Build history of the part. All positions in model axes, mm. A direction names the side the tool comes from. Round coordinates to 2 decimals unless told otherwise and drop trailing zeros. Loops run counter-clockwise (first coordinate to the right, second up) from the corner with the lowest first, then second, coordinate; pieces in that order, holes last.
from build123d import *

# Parameters (mm, degrees)
F1_DEPTH = 64.77
F4_DEPTH = 2.54
F5_DEPTH = 2.54
F6_R     = 2.667
F6_R_2   = 19.05
F7_DEPTH = 70.613
F9_DEPTH = 70.613


with BuildPart() as f1:
    # F0 (on Right) → F1 (new body)
    with BuildSketch(Plane.YZ):
        with BuildLine():
            Line((-58.708991, 56.24623), (-61.375991, 56.24623))
            Line((-61.375991, 56.24623), (-61.375991, -11.69877))
            Line((-61.375991, -11.69877), (-129.320991, -11.69877))
            Line((-129.320991, -11.69877), (-129.320991, -14.36577))
            Line((-129.320991, -14.36577), (-61.248991, -14.36577))
            ThreePointArc((-61.248991, -14.36577), (-59.45294, -13.621821), (-58.708991, -11.82577))
            Line((-58.708991, -11.82577), (-58.708991, 56.24623))
        make_face()
    extrude(amount=F1_DEPTH)

    # F3 (on face) → F4 (join)
    with BuildSketch(Plane(origin=(0, 0, 0), x_dir=(0, -1, 0), z_dir=(-1, 0, 0))):
        with BuildLine():
            Line((77.885991, -11.69877), (61.375991, 14.97123))
            Line((61.375991, 14.97123), (61.375991, -7.88877))
            ThreePointArc((61.375991, -7.88877), (62.491914, -10.582847), (65.185991, -11.69877))
            Line((65.185991, -11.69877), (77.885991, -11.69877))
        make_face()
    extrude(amount=-F4_DEPTH)

    # F2 (on face) → F5 (join)
    with BuildSketch(Plane.YZ.offset(64.77)):
        with BuildLine():
            Line((-61.375991, -7.88877), (-61.375991, 14.97123))
            Line((-61.375991, 14.97123), (-77.885991, -11.69877))
            Line((-77.885991, -11.69877), (-65.185991, -11.69877))
            ThreePointArc((-65.185991, -11.69877), (-62.491914, -10.582847), (-61.375991, -7.88877))
        make_face()
    extrude(amount=-F5_DEPTH)

    # F6 (on face) → F7 (cut, through all)
    with BuildSketch(Plane(origin=(0, -58.708991, 0), x_dir=(-1, 0, 0), z_dir=(0, 1, 0))):
        Polygon((-64.77, 56.24623), (-64.77, 49.89623), (-58.42, 56.24623), align=None)
        with Locations((-55.935, 51.03923)):
            Circle(F6_R)
        with Locations((-8.835, 51.03923)):
            Circle(F6_R)
        Polygon((0, 56.24623), (-6.35, 56.24623), (0, 49.89623), align=None)
        with Locations((-32.385, 27.48923)):
            Circle(F6_R_2)
        with Locations((-55.935, 3.93923)):
            Circle(F6_R)
        with Locations((-8.835, 3.93923)):
            Circle(F6_R)
    extrude(amount=-F7_DEPTH, mode=Mode.SUBTRACT)

    # F8 (on face) → F9 (cut, through all)
    with BuildSketch(Plane(origin=(0, 0, -14.36577), x_dir=(1, 0, 0), z_dir=(0, 0, -1))):
        Polygon((0, 129.320991), (0, 122.970991), (6.35, 129.320991), align=None)
        with BuildLine():
            Line((14.605, 77.885991), (14.605, 119.541991))
            ThreePointArc((14.605, 119.541991), (12.446, 121.700991), (10.287, 119.541991))
            Line((10.287, 119.541991), (10.287, 77.885991))
            ThreePointArc((10.287, 77.885991), (12.446, 75.726991), (14.605, 77.885991))
        make_face()
        with BuildLine():
            Line((54.483, 77.885991), (54.483, 119.541991))
            ThreePointArc((54.483, 119.541991), (52.324, 121.700991), (50.165, 119.541991))
            Line((50.165, 119.541991), (50.165, 77.885991))
            ThreePointArc((50.165, 77.885991), (52.324, 75.726991), (54.483, 77.885991))
        make_face()
        Polygon((64.77, 129.320991), (58.42, 129.320991), (64.77, 122.970991), align=None)
    extrude(amount=-F9_DEPTH, mode=Mode.SUBTRACT)


solid = f1.part
(1) Slice it at B-B on x = 32. List the corners of the cut face in (y, z), plus the area to 3 significant figures.
Responses:
outline: (-129.32, -14.37) - (-61.25, -14.37) arc R2.54 ccw to (-58.71, -11.83) - (-58.71, 8.44) - (-61.38, 8.44) - (-61.38, -11.7) - (-129.32, -11.7) - close; (-61.38, 46.54) - (-58.71, 46.54) - (-58.71, 56.25) - (-61.38, 56.25) - close
area: 267 mm2
(2) Slice it at A-A on y = -117.5. List the corners of the cut face in (x, z) (3 decimals).
Responses:
outline: (0, -14.366) - (10.287, -14.366) - (10.287, -11.699) - (0, -11.699) - close; (14.605, -14.366) - (50.165, -14.366) - (50.165, -11.699) - (14.605, -11.699) - close; (54.483, -14.366) - (64.77, -14.366) - (64.77, -11.699) - (54.483, -11.699) - close
(3) Which spindle directions (+Z, -Z, +X, -X, +Y, -Y) get a long thin tool onto all of the face, cutting with end or side? Do faces 1 (the face through (63.518, -69.515, 1.823)), 2 (the face through (12.399, -75.728, -13.051)), 3 (the face through (2.54, -66, -4)). Say none if no direction does.
Responses:
face 1: +Z, +X, -X, -Y
face 2: +Z, -Z
face 3: +Z, -Y
(4) Slice it at D-D on x = 8.5. List the corners of the cut face in (y, z).
Responses:
outline: (-129.32, -14.37) - (-61.25, -14.37) arc R2.54 ccw to (-58.71, -11.83) - (-58.71, 1.29) - (-61.38, 1.29) - (-61.38, -11.7) - (-129.32, -11.7) - close; (-61.38, 6.59) - (-58.71, 6.59) - (-58.71, 48.39) - (-61.38, 48.39) - close; (-61.38, 53.69) - (-58.71, 53.69) - (-58.71, 56.25) - (-61.38, 56.25) - close
(5) Pull direction Z, two halves, no side cores. Call faces 4 (the face through (52.277, -75.728, -13.051)), 5 (the face through (32, -96, -14.366)), 6 (the face through (46.43, -60.02, 40.36)), 7 (the face through (61.639, -60.024, 53.027)): +Z half, -Z half, draft (parallel to the pull), parting line (faces both ways), or undercut.
Responses:
face 4: draft
face 5: -Z half
face 6: undercut
face 7: +Z half
(6) Pin check, flat tips, straight feed: P1, Ø19.5, axis at x = 27.5, z = 30, coming from the -Y side; P2, Ø19.5, axis at x = 21.5, y = -104.5, coming from the +Z side; P3, Ø6, axis at x = 10.5, z = 38.5, coming from the -Y side. Stop position of each tip, or through.
Responses:
P1: passes through
P2: stops at z = -11.7
P3: stops at y = -61.38
(7) Probe line 1 (X direction, y = -66, z = -4.5); line 2 (Y direction, x = 56, z = -9.5); line 3 (Z direction, x = 45, y = -123.5). List the from-to ranges inside material, lowest first.
Responses:
line 1: x = 0 to 2.54, 62.23 to 64.77
line 2: y = -61.38 to -58.71
line 3: z = -14.37 to -11.7
(8) Slice it at C-C on z = 18.5. List the corners of the cut face in (x, y), plus the area to 3 significant figures.
Responses:
outline: (0, -61.38) - (15.59, -61.38) - (15.59, -58.71) - (0, -58.71) - close; (49.18, -61.38) - (64.77, -61.38) - (64.77, -58.71) - (49.18, -58.71) - close
area: 83.2 mm2
